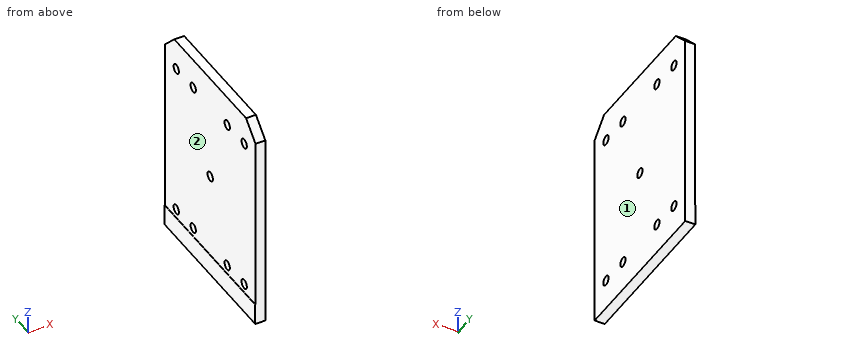
from build123d import *

# Parameters (mm, degrees)
F1_DEPTH = 19.05
F2_R     = 8.89
F3_DEPTH = 96.012
F4_W     = 304.8
F4_H     = 366.342949
F5_DEPTH = 0.508


with BuildPart() as f1:
    # F0 (on Right) → F1 (new body)
    with BuildSketch(Plane.YZ):
        Polygon((-152.4, -203.2), (152.4, -203.2), (152.4, 171.45), (120.65, 203.2), (-120.65, 203.2), (-152.4, 171.45), align=None)
    extrude(amount=F1_DEPTH)

    # F2 (on face) → F3 (cut)
    with BuildSketch(Plane.YZ.offset(19.05)):
        with Locations((-57.15, 146.000296)):
            Circle(F2_R)
        with Locations((-114.3, 146.000296)):
            Circle(F2_R)
        Circle(F2_R)
        with Locations((-57.15, -146.000296)):
            Circle(F2_R)
        with Locations((-114.3, -146.000296)):
            Circle(F2_R)
        with Locations((57.15, 146.000296)):
            Circle(F2_R)
        with Locations((114.3, 146.000296)):
            Circle(F2_R)
        with Locations((57.15, -146.000296)):
            Circle(F2_R)
        with Locations((114.3, -146.000296)):
            Circle(F2_R)
    extrude(amount=-F3_DEPTH, mode=Mode.SUBTRACT)

    # F4 (on face) → F5 (cut)
    with BuildSketch(Plane(origin=(0, 0, 0), x_dir=(0, -1, 0), z_dir=(-1, 0, 0))):
        with Locations((0, 20.028526)):
            Rectangle(F4_W, F4_H)
    extrude(amount=-F5_DEPTH, mode=Mode.SUBTRACT)


solid = f1.part
Work out the finished part from the listing and answer in its coordinate system (mm). Face numbers are marked on the shaded views. A direction names the side the tool comes from. Round coordinates to 2 decimals unless told otherwise and drop trailing zeros. Write each loop counter-clockwise with the first axis right and the second up, starting at its lowest first coordinate (ties: lowest second). Pieces come first, ordered by that corner, then holes. Notation, with made-up numbers: M -17,9 L 28,9 A19 ccw 28,28 Z; hole C -4.75,-15.75 d4. An arc over 180 degrees is marked long. Use a Markdown table: item, result.
1) The part is cut by section A-A on y = 0. Give the vertices of the cut face in (x, z), plus the area to 3 significant figures.
Taken from the geometry:
| item | result |
|---|---|
| outline | M 0,-203.2 L 19.05,-203.2 L 19.05,-8.89 L 0.51,-8.89 L 0.51,-163.14 L 0,-163.14 Z; M 0.51,8.89 L 19.05,8.89 L 19.05,203.2 L 0.51,203.2 Z |
| area | 7,230 mm2 |
2) Flat-ended cylindrical pins translate along their axes: pin 1 (14 mm diameter, centred on y = -114.3, z = -146, fed in from -X); pin 2 (1 mm diameter, centred on y = 57.5, z = 87, fed in from -X). Find the tip coordinate at first contact, or state that the pin passes through.
Taken from the geometry:
| item | result |
|---|---|
| pin 1 | passes through |
| pin 2 | stops at x = 0.51 |
3) The part is cut by section D-D on z = 98. Give the vertices of the cut face in (x, y), plus the area to 3 significant figures.
Taken from the geometry:
| item | result |
|---|---|
| outline | M 0.51,-152.4 L 19.05,-152.4 L 19.05,152.4 L 0.51,152.4 Z |
| area | 5,650 mm2 |
4) Consider line 1 (Z direction, x = 17, y = 113); line 2 (Z direction, x = 5.75, y = -57.15); line 3 (Y direction, x = 18, z = 145.5). Determine where each line is inside the solid, lowest interval first. Write a range as [from, to].
Taken from the geometry:
| item | result |
|---|---|
| line 1 | z = [-203.2, -154.79], [-137.21, 137.21], [154.79, 203.2] |
| line 2 | z = [-203.2, -154.89], [-137.11, 137.11], [154.89, 203.2] |
| line 3 | y = [-152.4, -123.18], [-105.42, -66.03], [-48.27, 48.27], [66.03, 105.42], [123.18, 152.4] |
5) Which of the six approach directions +Z, -Z, +X, -X, +Y, -Y give full straight-line access (tool end or side, diameter ignored) to the marked faces 1 and 2?
Taken from the geometry:
| item | result |
|---|---|
| face 1 | +Z, -Z, +X, +Y, -Y |
| face 2 | +Z, -X, +Y, -Y |
6) The part is cut by section B-B on x = 7. State how many separate pieces and enclosed holes the cut face has, plus the area to 3 significant figures.
Taken from the geometry:
| item | result |
|---|---|
| separate pieces | 1 |
| enclosed holes | 9 |
| area | 121,000 mm2 |
7) The part is cut by section C-C on y = 114.3. Give the vertices of the cut face in (x, z).
Taken from the geometry:
| item | result |
|---|---|
| outline | M 0,-203.2 L 19.05,-203.2 L 19.05,-154.89 L 0.51,-154.89 L 0.51,-163.14 L 0,-163.14 Z; M 0.51,-137.11 L 19.05,-137.11 L 19.05,137.11 L 0.51,137.11 Z; M 0.51,154.89 L 19.05,154.89 L 19.05,203.2 L 0.51,203.2 Z |
